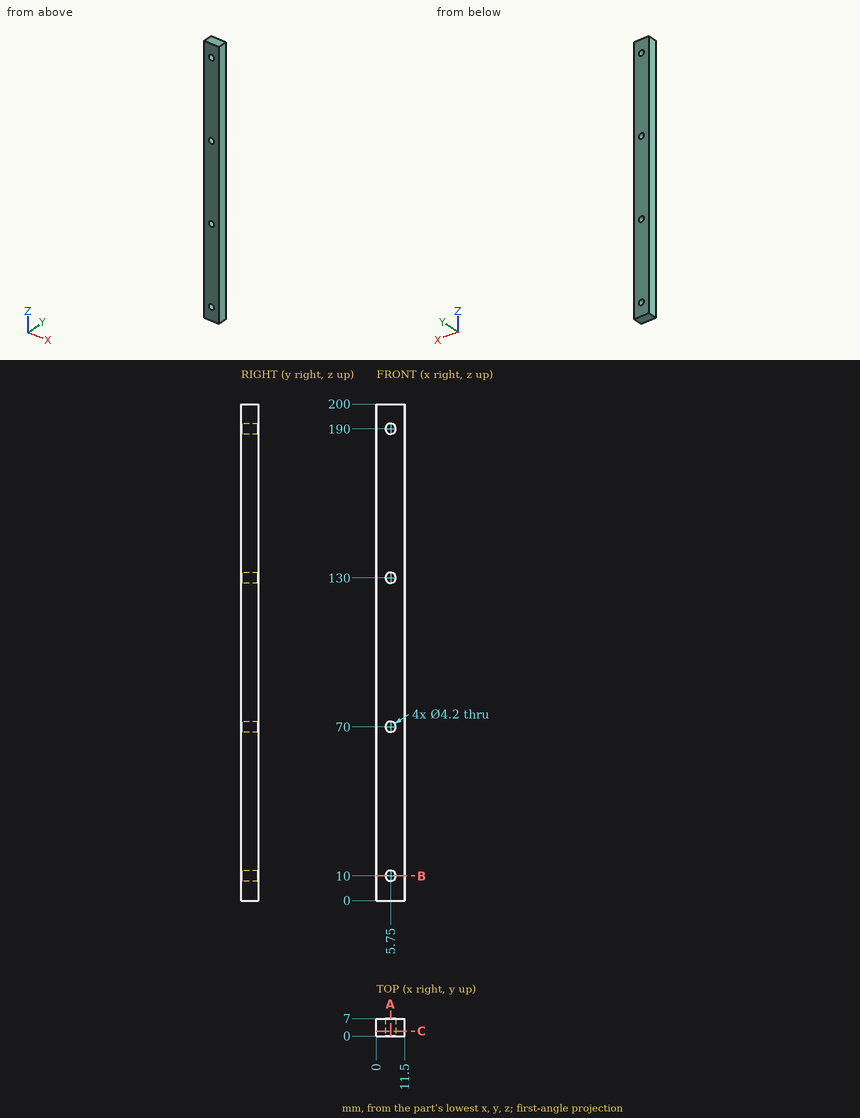
The figure shows three views and two pictorial views of one solid part (mm, origin at its lowest corner). Answer the questions. Give positions to 0.01 mm unless a question says otherwise; leave off trailing zeros. Order: outer loops, then holes, each group sorted by start corner. A loop starts at its lowest first (then second) coordinate and runs counter-clockwise, first axis right, second up. Notation, with made-up numbers: M 72.25,78.5 L 80.25,78.5 A13 ccw 80.25,100.5 Z; hole C -36.5,1.25 d2. An arc over 180 degrees is marked long. Return JSON: item names as keys, results as strings.
Q1. Find section C-C, the plane y = 2. Write down the section's boundary in (x, z).
Answer below:
{"outline": "M 0,0 L 11.5,0 L 11.5,200 L 0,200 Z; hole C 5.75,10 d4.2; hole C 5.75,70 d4.2; hole C 5.75,130 d4.2; hole C 5.75,190 d4.2"}
Q2. Find section B-B, the plane z = 10. Write down the section's boundary in (x, y), and give its area (3 significant figures).
Answer below:
{"outline": "M 0,0 L 3.65,0 L 3.65,7 L 0,7 Z; M 7.85,0 L 11.5,0 L 11.5,7 L 7.85,7 Z", "area": "51.1 mm^2"}
Q3. Find the intervals of material crossed by line 1 along Z through (x, y) = (5.75, 3.5); line 2 along X through (y, z) = (3, 70); line 3 along Z through (x, y) = (7.5, 0.75), in increasing order. Write a range as [from, to].
Answer below:
{"line 1": "z = [0, 7.9], [12.1, 67.9], [72.1, 127.9], [132.1, 187.9], [192.1, 200]", "line 2": "x = [0, 3.65], [7.85, 11.5]", "line 3": "z = [0, 8.84], [11.16, 68.84], [71.16, 128.84], [131.16, 188.84], [191.16, 200]"}
Q4. This flat-tipped pin is pushed along its axis until it touches: pin 1 (5 mm diameter, centred on x = 5.75, z = 10, fed in from +Y). Where does it stop, or does it pass through?
Answer below:
{"pin 1": "stops at y = 7"}
Q5. Find section A-A, the plane x = 5.75. Write down the section's boundary in (y, z), and give its area (3 significant figures).
Answer below:
{"outline": "M 0,0 L 7,0 L 7,7.9 L 0,7.9 Z; M 0,12.1 L 7,12.1 L 7,67.9 L 0,67.9 Z; M 0,72.1 L 7,72.1 L 7,127.9 L 0,127.9 Z; M 0,132.1 L 7,132.1 L 7,187.9 L 0,187.9 Z; M 0,192.1 L 7,192.1 L 7,200 L 0,200 Z", "area": "1,280 mm^2"}
